Model file for the job. Use its own axes, mm. A direction names the side the tool comes from. Coordinates: 2 decimals unless noted, no trailing zeros. Write each loop counter-clockwise with the first axis right and the second up, starting at its lowest first coordinate (ties: lowest second). Pieces come first, ordered by that corner, then holes.
Q1. Which spindle directions (+Z, -Z, +X, -X, +Y, -Y) get a long thin tool onto all of the face, cutting with end or side? Do faces 4 (the cylindrical face through (23.664, 3.685, -12.851)), 5 (the flat face through (24, -2, -8)), 6 (the cylindrical face through (23.66, 4.99, -10.1)). Say none if no direction does.
Q2. Band-saw the part on A-A, the plane z = -21.5. Write the cut outline in (x, y), plus the area to 3 significant figures.
Q3. Pull direction Z, two halves, no side cores. Call faces 1 (the flat face through (24, -34, -17)), 2 (the cylindrical face through (23.66, 3.15, -32.89)), 3 (the flat face through (24, -14, -35.9)): released by +Z, released by -Z, zero draft, split by the parting line, or undercut.
Q4. Pin check, flat tips, straight feed: P1, Ø4, axis at x = 33.5, y = -15.5, coming from the +Z side; P2, Ø3, axis at x = 14, z = -12, coming from the +Y side; P3, Ø3, axis at x = 28, y = -27, coming from the +Z side. Stop position of each tip, or through.
Q5. Band-saw the part on D-D, the plane y = -16. Write the cut outline in (x, z), plus the area to 3 significant figures.
Q6. Band-saw the part on B-B, the plane y = 3.5. Write the cut outline in (x, z).
Q7. Drill centre lines: probe 1 along Y at (x, z) = (17, -20); probe 2 along Z at (x, y) = (14.5, -10.5); probe 3 along Y at (x, z) = (29, -13). Where is each one in solid material? Low to high.
Q8. Band-saw the part on C-C, the plane x = 29. Write the cut outline in (y, z).
from build123d import *

# Parameters (mm, degrees)
BOSS_EXTRUDE3_DEPTH = 48
CUT_EXTRUDE2_DEPTH  = 54


with BuildPart() as part:
    # Sketch3 → Boss-Extrude3 (new body)
    with BuildSketch(Plane(origin=(0, 0, 0), x_dir=(0, 0, -1), z_dir=(1, 0, 0))):
        with BuildLine():
            Line((7.25, -20.3), (7.25, -11.034312351))
            Line((7.25, -11.034312351), (7.25, -2))
            ThreePointArc((7.25, -2), (10.178932188, 5.071067812), (17.25, 8))
            Line((17.25, 8), (27.9, 8))
            ThreePointArc((27.9, 8), (34.971067812, 5.071067812), (37.9, -2))
            Line((37.9, -2), (37.9, -20.3))
            Line((37.9, -20.3), (37.9, -36))
            Line((37.9, -36), (7.25, -36))
            Line((7.25, -36), (7.25, -20.3))
        make_face()
        with BuildLine():
            Line((9.25, -20.3), (9.25, -11.034312351))
            Line((9.25, -11.034312351), (9.25, -4))
            ThreePointArc((9.25, -4), (12.178932188, 3.071067812), (19.25, 6))
            Line((19.25, 6), (25.9, 6))
            ThreePointArc((25.9, 6), (32.971067812, 3.071067812), (35.9, -4))
            Line((35.9, -4), (35.9, -20.3))
            Line((35.9, -20.3), (35.9, -24))
            ThreePointArc((35.9, -24), (32.971067812, -31.071067812), (25.9, -34))
            Line((25.9, -34), (9.25, -34))
            Line((9.25, -34), (9.25, -20.3))
        make_face(mode=Mode.SUBTRACT)
    extrude(amount=BOSS_EXTRUDE3_DEPTH)

    # Sketch4 → Cut-Extrude2 (cut)
    with BuildSketch(Plane.ZY):
        Polygon((-9.25, -34), (-7.25, -34), (-7.25, -2), (-9.452041029, -2), align=None)
    extrude(amount=-CUT_EXTRUDE2_DEPTH, mode=Mode.SUBTRACT)


solid = part.part
Answer sheet:
1. face 4: +X, -X
1. face 5: +Z, +X, -X
1. face 6: +Z, +X, -X, +Y
2. outline: (0, -36) - (48, -36) - (48, -34) - (0, -34) - close; (0, 6) - (48, 6) - (48, 8) - (0, 8) - close
2. area: 192 mm2
3. face 1: zero draft
3. face 2: undercut
3. face 3: released by +Z
4. P1: stops at z = -35.9
4. P2: stops at y = 7.27
4. P3: stops at z = -34.83
5. outline: (0, -37.9) - (48, -37.9) - (48, -35.9) - (0, -35.9) - close
5. area: 96.0 mm2
6. outline: (0, -36.25) - (48, -36.25) - (48, -32.51) - (0, -32.51) - close; (0, -12.64) - (48, -12.64) - (48, -8.9) - (0, -8.9) - close
7. probe 1: y = -36 to -34, 6 to 8
7. probe 2: z = -37.9 to -35.9
7. probe 3: y = -36 to -34, 3.81 to 7.05
8. outline: (-36, -37.9) - (-2, -37.9) arc R10 ccw to (8, -27.9) - (8, -17.25) arc R10 ccw to (-2, -7.25) - (-2, -9.45) arc R10 cw to (6, -19.25) - (6, -25.9) arc R10 cw to (-4, -35.9) - (-24, -35.9) arc R10 cw to (-34, -25.9) - (-34, -7.25) - (-36, -7.25) - close
